Can you work these out from the model? Positions are in its coordinate system, mm. A direction names the side the tool comes from. Give positions to 0.01 mm unless a question says otherwise; leave off trailing zeros. Write each loop counter-clockwise with the first axis right and the second up, starting at its lowest first coordinate (ties: lowest second). Pieces come first, ordered by that corner, then holes. Notation, with made-up numbers: (88, 21.25) -> (135, 21.25) arc R19 ccw to (135, 31.25) -> close; hole circle Ø10 at (83, 7.5). An arc over 180 degrees is marked (long way). One line per item, written item: value.
Autodesk Inventor part; units mm, degrees
ref_plane "YZ Plane" through (0, 0, 0) normal (1, 0, 0) x (0, 1, 0)
ref_plane "XZ Plane" through (0, 0, 0) normal (0, 1, 0) x (-1, 0, 0)
ref_plane "XY Plane" through (0, 0, 0) normal (0, 0, 1) x (1, 0, 0)
sketch "Sketch1" plane through (0, 0, 0) normal (0, 1, 0) x (-1, 0, 0)
  circle A0 centre (0, 0) radius 18.6309
  dimension "d0" = 37.2618
extrude "Extrusion1" add sketch "Sketch1" along normal blind 57.0738
sketch "Sketch2" plane through (0, 57.0738, 0) normal (0, 1, 0) x (1, 0, 0)
  circle A0 centre (0, 0) radius 6.604
  dimension "d3" = 13.208
extrude "Extrusion2" add sketch "Sketch2" along normal blind 5.08
sketch "Sketch3" plane through (0, 57.0738, 0) normal (0, 1, 0) x (1, 0, 0)
  circle A0 centre (0, 13.5382) radius 1.27
  circle A1 centre (0, -13.5382) radius 1.2719
  circle A2 centre (14.8082, 0) radius 1.27
  point P0 (0, 0)
  dimension "d6" = 2.54
  dimension "d7" = 2.54
  dimension "d8" = 13.5382
  dimension "d9" = 13.5382
  dimension "d10" = 14.8082
extrude "Extrusion3" cut sketch "Sketch3" against normal blind 76.2
sketch "Sketch4" plane through (0, 62.1538, 0) normal (0, 1, 0) x (1, 0, 0)
  circle A0 centre (0, 0) radius 1.7145
  dimension "d13" = 3.429
extrude "Extrusion4" add sketch "Sketch4" along normal blind 12.7
sketch "Sketch5" plane through (0, 74.8538, 0) normal (0, 1, 0) x (1, 0, 0)
  point P0 (0, 0)
properties part number "motor MABCHI 3W Noah"
1) If we section it at D-D (z = -5): Write out the boundary of the cut face in (x, y), and give its area (3 significant figures).
Answer list:
outline: (-17.95, 0) -> (17.95, 0) -> (17.95, 57.07) -> (4.31, 57.07) -> (4.31, 62.15) -> (-4.31, 62.15) -> (-4.31, 57.07) -> (-17.95, 57.07) -> close
area: 2,090 mm^2
2) If we section it at B-B (x = 0): Write out the boundary of the cut face in (y, z).
Answer list:
outline: (0, -18.63) -> (57.07, -18.63) -> (57.07, -14.81) -> (0, -14.81) -> close; (0, -12.27) -> (57.07, -12.27) -> (57.07, -6.6) -> (62.15, -6.6) -> (62.15, -1.71) -> (74.85, -1.71) -> (74.85, 1.71) -> (62.15, 1.71) -> (62.15, 6.6) -> (57.07, 6.6) -> (57.07, 12.27) -> (0, 12.27) -> close; (0, 14.81) -> (57.07, 14.81) -> (57.07, 18.63) -> (0, 18.63) -> close
3) If we section it at C-C (x = -4): Write out the boundary of the cut face in (y, z), and give its area (3 significant figures).
Answer list:
outline: (0, -18.2) -> (57.07, -18.2) -> (57.07, -5.25) -> (62.15, -5.25) -> (62.15, 5.25) -> (57.07, 5.25) -> (57.07, 18.2) -> (0, 18.2) -> close
area: 2,130 mm^2
4) I need wall thicknesses on L1, parallel to Z at x = 0, y = 38.5; L2, parallel to Y at x = -10.5, z = -5.5; L3, parallel to Y at x = 5, z = -1. Which ranges of each line are inside material? Lowest first, please.
Answer list:
L1: z = -18.63 to -14.81, -12.27 to 12.27, 14.81 to 18.63
L2: y = 0 to 57.07
L3: y = 0 to 62.15
5) If we section it at A-A (z = 0): Write out the boundary of the cut face in (x, y), and give its area (3 significant figures).
Answer list:
outline: (-18.63, 0) -> (13.54, 0) -> (13.54, 57.07) -> (6.6, 57.07) -> (6.6, 62.15) -> (1.71, 62.15) -> (1.71, 74.85) -> (-1.71, 74.85) -> (-1.71, 62.15) -> (-6.6, 62.15) -> (-6.6, 57.07) -> (-18.63, 57.07) -> close; (16.08, 0) -> (18.63, 0) -> (18.63, 57.07) -> (16.08, 57.07) -> close
area: 2,090 mm^2
6) For faces 1 (the face through (-17.77, 28.14, -5.6)), 2 (the face through (0, 57.074, -8)), which set-ups out of +Z, -Z, +X, -X, +Y, -Y let a thin tool reach every point of the face, with its end or its side?
Answer list:
face 1: +Y, -Y
face 2: +Y
7) Will these pins go through, and if not, where does the flat tip stop? pin 1 (2 mm diameter, centred on y = 59, z = -6.5, fed in from +X); pin 2 (6 mm diameter, centred on x = 10.5, y = 21, fed in from -Z); pin 3 (5 mm diameter, centred on x = -13, y = 32.5, fed in from +Z); pin 4 (12 mm diameter, centred on y = 34, z = -4, fed in from +X).
Answer list:
pin 1: stops at x = 3.66
pin 2: stops at z = -17.05
pin 3: stops at z = 15.39
pin 4: stops at x = 18.63
